Here's the drawing with two shaded views (mm, measured from the low corner). I have some questions. Round coordinates to 2 decimals unless told otherwise and drop trailing zeros. Loops run counter-clockwise (first coordinate to the right, second up) from the corner with the lowest first, then second, coordinate; pieces in that order, holes last. Notation, with made-up numbers: (11, -22.5) - (66, -22.5) arc R35 ccw to (66, 12.5) - close; hole circle Ø5 at (22.5, 55.5). An arc over 180 degrees is marked (long way). Use one line per item in the form item = value.
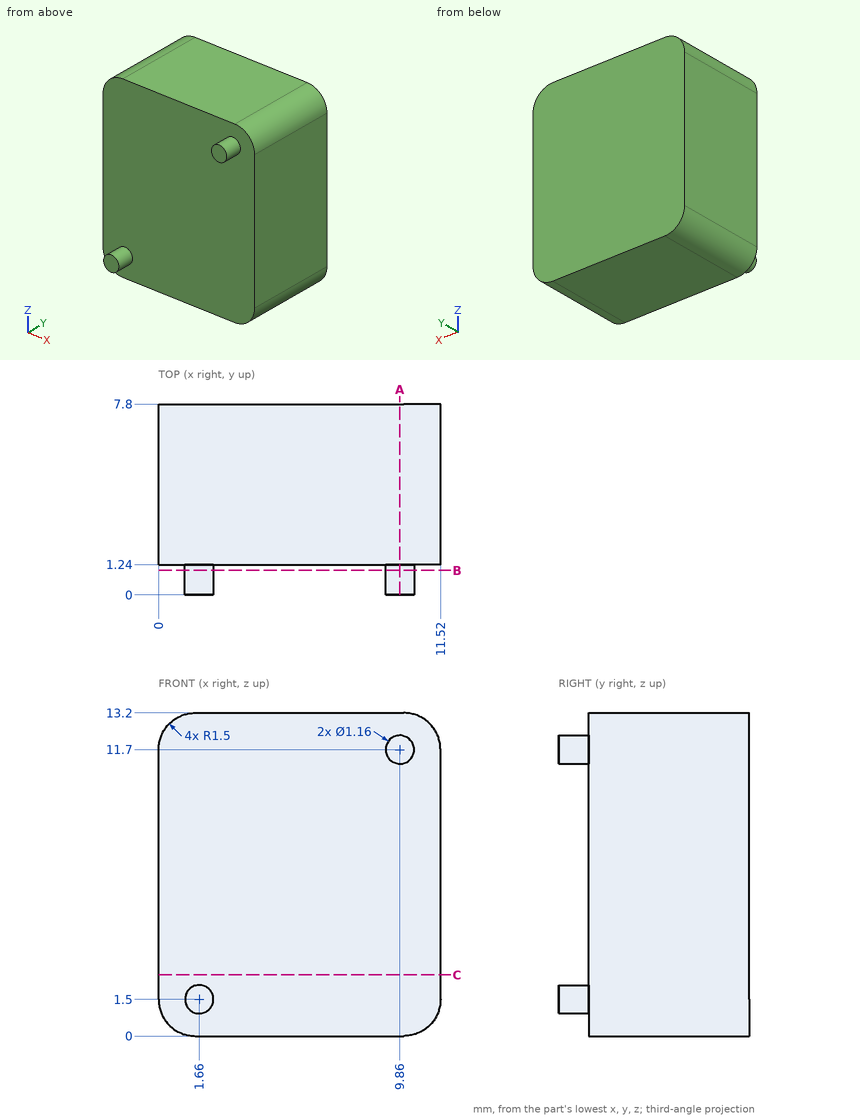
1. Please list where these lines run through material, in increasing order: line 1 along Y through (x, z) = (7, 12.5); line 2 along Z through (x, y) = (9.5, 1); line 3 along Z through (x, y) = (10.5, 7).
Solution:
line_1 = 1.24 to 7.8
line_2 = 11.25 to 12.15
line_3 = 0.08 to 13.12
2. If we section it at C-C, the plane z = 2.5: Write out the boundary of the cut face in (x, y), plus the area to 3 significant figures.
Solution:
outline = (0, 1.24) - (11.52, 1.24) - (11.52, 7.8) - (0, 7.8) - close
area = 75.6 mm^2
3. For P1, Ø3.5, axis at x = 7, z = 6, coming from the -Y side, with a flat end and sliding along its axis, tell me the tip position at first contact or that it passes through.
Solution:
P1 = 1.24
4. If we section it at A-A, the plane x = 9.86: Write out the boundary of the cut face in (y, z).
Solution:
outline = (0, 11.12) - (1.24, 11.12) - (1.24, 0) - (7.8, 0) - (7.8, 13.2) - (1.24, 13.2) - (1.24, 12.28) - (0, 12.28) - close
5. If we section it at B-B, the plane y = 1: Write out the boundary of the cut face in (x, z), plus the area to 3 significant figures.
Solution:
outline = circle Ø1.16 at (1.66, 1.5); circle Ø1.16 at (9.86, 11.7)
area = 2.11 mm^2
